Check sheet for the drawn part. Datum: minimum x, y, z corner. Units: mm. A direction names the side the tool comes from. Coordinates: 2 decimals unless noted, no trailing zeros. Loops run counter-clockwise (first coordinate to the right, second up) from the corner with the lowest first, then second, coordinate; pieces in that order, holes last.
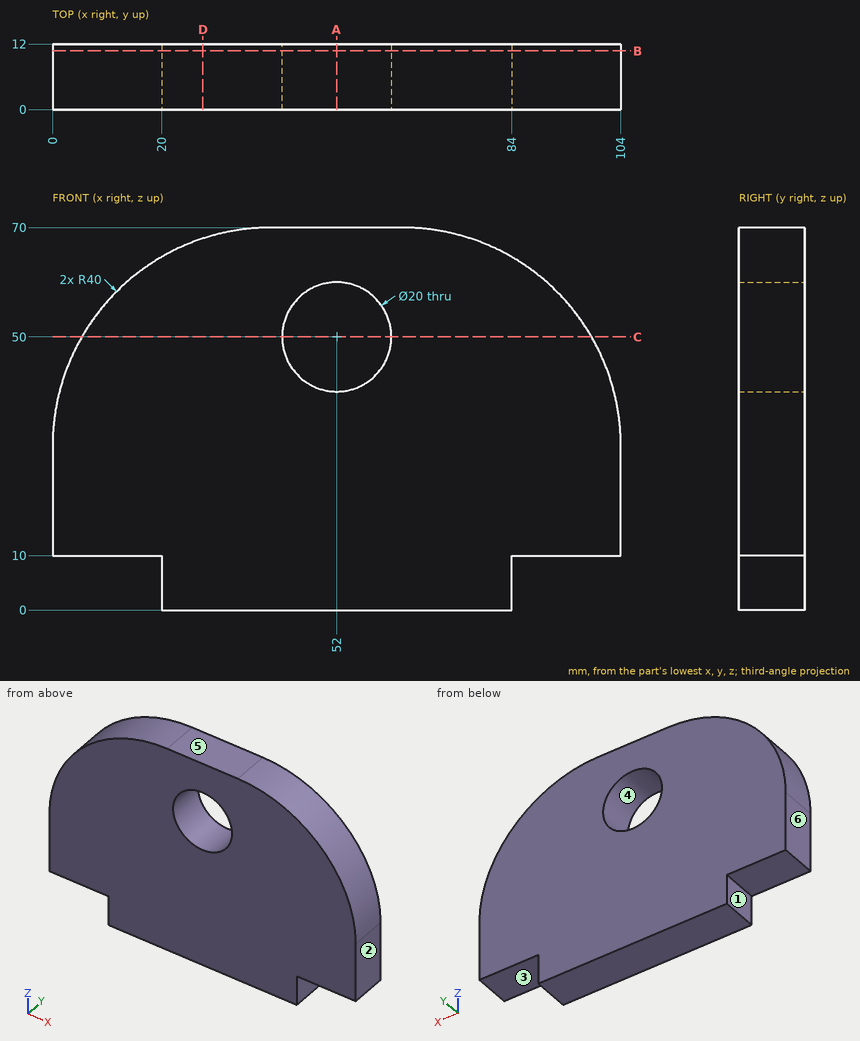
(1) Sectioned sample at C-C on z = 50. Record the cut outline in (x, y).
Findings:
outline: (5.36, 0) - (42, 0) - (42, 12) - (5.36, 12) - close; (62, 0) - (98.64, 0) - (98.64, 12) - (62, 12) - close
(2) Gauge pin test, flat ends, axial feed: pin 1 Ø1 at (y, z) = (7, 40) entering from -X; pin 2 Ø3 at (y, z) = (6.5, 7) entering from +X; pin 3 Ø3 at (y, z) = (5, 3.5) entering from -X. Record the tip position at first contact, or that the pin passes through.
Findings:
pin 1: stops at x = 1.14
pin 2: stops at x = 84
pin 3: stops at x = 20
(3) Sectioned sample at D-D on x = 27.5. Record the cut outline in (y, z).
Findings:
outline: (0, 0) - (12, 0) - (12, 68) - (0, 68) - close
(4) Draft check along Z on the marked faces 3, 4, 5 and 6. Enter one of: +Z half, -Z half, draft (parallel to the pull), parting line (faces both ways), or undercut.
Findings:
face 3: -Z half
face 4: undercut
face 5: +Z half
face 6: draft
(5) Sectioned sample at A-A on x = 52. Record the cut outline in (y, z), and give its area (3 significant figures).
Findings:
outline: (0, 0) - (12, 0) - (12, 40) - (0, 40) - close; (0, 60) - (12, 60) - (12, 70) - (0, 70) - close
area: 600 mm2
(6) Sectioned sample at B-B on y = 10.75. Record the cut outline in (x, z).
Findings:
outline: (0, 10) - (20, 10) - (20, 0) - (84, 0) - (84, 10) - (104, 10) - (104, 30) arc R40 ccw to (64, 70) - (40, 70) arc R40 ccw to (0, 30) - close; hole circle Ø20 at (52, 50)
(7) Access from +Z, -Z, +X, -X, +Y, -Y to the whole of each face (thin tool, end or side, straight path). Record for the marked faces 1 and 2.
Findings:
face 1: -Z, -X, +Y, -Y
face 2: +Z, -Z, +X, +Y, -Y
(8) Scan lines: L1, parallel to Z at x = 52, y = 9.5; L2, parallel to X at y = 7.5, z = 5; L3, parallel to Z at x = 68, y = 6.5. Record each from-to range of solid material in increasing order.
Findings:
L1: z = 0 to 40, 60 to 70
L2: x = 20 to 84
L3: z = 0 to 69.8
